CAD build for the part. Positions are in the model's coordinates, mm. Give positions to 0.01 mm unless a question says otherwise; leave off trailing zeros. Put each result on its own line as item: value. Start each with the question number.
1. Drop flat-ended pins along their axis: pin 1 (2 mm diameter, centred on y = -38, z = -75.5, fed in from -X); pin 2 (5 mm diameter, centred on y = -21.5, z = -175.5, fed in from -X); pin 3 (2.5 mm diameter, centred on x = 0, y = -20, fed in from -Z); pin 4 (1.3 mm diameter, centred on x = 1.5, z = -241.5, fed in from -Y). Give the stop position or say it passes through.
2. Cut at A-A on z = -411.5. Give the number of separate pieces and of enclosed holes in the cut face, and give its area (3 significant figures).
3. Wall check: line 1 (Y direction, x = 0, z = -257); line 2 (Y direction, x = -0.5, z = -439.5); line 3 (Y direction, x = 2.5, z = -181). Give the ranges that are in metal, low to high.
from build123d import *

# Parameters (mm, degrees)
SKETCH2_R           = 2.1
BOSS_EXTRUDE2_DEPTH = 500


with BuildPart() as part:
    # Sketch2 → Boss-Extrude2 (new body)
    with BuildSketch(Plane.XY):
        with BuildLine():
            Line((-9.5, 10), (-4.58, 10))
            Line((-4.58, 10), (-3.13, 8.55))
            Line((-3.13, 8.55), (-3.13, 8.2))
            Line((-3.13, 8.2), (-5.5, 8.2))
            Line((-5.5, 8.2), (-5.5, 6.56))
            Line((-5.5, 6.56), (-2.84, 3.9))
            Line((-2.84, 3.9), (-0.21, 3.9))
            Line((-0.21, 3.9), (0, 3.69))
            Line((0, 3.69), (0.21, 3.9))
            Line((0.21, 3.9), (2.84, 3.9))
            Line((2.84, 3.9), (5.5, 6.56))
            Line((5.5, 6.56), (5.5, 8.2))
            Line((5.5, 8.2), (3.13, 8.2))
            Line((3.13, 8.2), (3.13, 8.55))
            Line((3.13, 8.55), (4.58, 10))
            Line((4.58, 10), (9.5, 10))
            ThreePointArc((9.5, 10), (9.853553391, 9.853553391), (10, 9.5))
            Line((10, 9.5), (10, 4.58))
            Line((10, 4.58), (8.55, 3.13))
            Line((8.55, 3.13), (8.2, 3.13))
            Line((8.2, 3.13), (8.2, 5.5))
            Line((8.2, 5.5), (6.56, 5.5))
            Line((6.56, 5.5), (3.9, 2.84))
            Line((3.9, 2.84), (3.9, 0.21))
            Line((3.9, 0.21), (3.69, 0))
            Line((3.69, 0), (3.9, -0.21))
            Line((3.9, -0.21), (3.9, -2.84))
            Line((3.9, -2.84), (6.56, -5.5))
            Line((6.56, -5.5), (8.2, -5.5))
            Line((8.2, -5.5), (8.2, -3.13))
            Line((8.2, -3.13), (8.55, -3.13))
            Line((8.55, -3.13), (10, -4.58))
            Line((10, -4.58), (10, -10))
            Line((10, -10), (10, -15.42))
            Line((10, -15.42), (8.55, -16.87))
            Line((8.55, -16.87), (8.2, -16.87))
            Line((8.2, -16.87), (8.2, -14.5))
            Line((8.2, -14.5), (6.56, -14.5))
            Line((6.56, -14.5), (3.9, -17.16))
            Line((3.9, -17.16), (3.9, -19.79))
            Line((3.9, -19.79), (3.69, -20))
            Line((3.69, -20), (3.9, -20.21))
            Line((3.9, -20.21), (3.9, -22.84))
            Line((3.9, -22.84), (6.56, -25.5))
            Line((6.56, -25.5), (8.2, -25.5))
            Line((8.2, -25.5), (8.2, -23.13))
            Line((8.2, -23.13), (8.55, -23.13))
            Line((8.55, -23.13), (10, -24.58))
            Line((10, -24.58), (10, -30))
            Line((10, -30), (10, -35.42))
            Line((10, -35.42), (8.55, -36.87))
            Line((8.55, -36.87), (8.2, -36.87))
            Line((8.2, -36.87), (8.2, -34.5))
            Line((8.2, -34.5), (6.56, -34.5))
            Line((6.56, -34.5), (3.9, -37.16))
            Line((3.9, -37.16), (3.9, -39.79))
            Line((3.9, -39.79), (3.69, -40))
            Line((3.69, -40), (3.9, -40.21))
            Line((3.9, -40.21), (3.9, -42.84))
            Line((3.9, -42.84), (6.56, -45.5))
            Line((6.56, -45.5), (8.2, -45.5))
            Line((8.2, -45.5), (8.2, -43.13))
            Line((8.2, -43.13), (8.55, -43.13))
            Line((8.55, -43.13), (10, -44.58))
            Line((10, -44.58), (10, -49.5))
            ThreePointArc((10, -49.5), (9.853553391, -49.853553391), (9.5, -50))
            Line((9.5, -50), (4.58, -50))
            Line((4.58, -50), (3.13, -48.55))
            Line((3.13, -48.55), (3.13, -48.2))
            Line((3.13, -48.2), (5.5, -48.2))
            Line((5.5, -48.2), (5.5, -46.56))
            Line((5.5, -46.56), (2.84, -43.9))
            Line((2.84, -43.9), (0.21, -43.9))
            Line((0.21, -43.9), (0, -43.69))
            Line((0, -43.69), (-0.21, -43.9))
            Line((-0.21, -43.9), (-2.84, -43.9))
            Line((-2.84, -43.9), (-5.5, -46.56))
            Line((-5.5, -46.56), (-5.5, -48.2))
            Line((-5.5, -48.2), (-3.13, -48.2))
            Line((-3.13, -48.2), (-3.13, -48.55))
            Line((-3.13, -48.55), (-4.58, -50))
            Line((-4.58, -50), (-9.5, -50))
            ThreePointArc((-9.5, -50), (-9.853553391, -49.853553391), (-10, -49.5))
            Line((-10, -49.5), (-10, -44.58))
            Line((-10, -44.58), (-8.55, -43.13))
            Line((-8.55, -43.13), (-8.2, -43.13))
            Line((-8.2, -43.13), (-8.2, -45.5))
            Line((-8.2, -45.5), (-6.56, -45.5))
            Line((-6.56, -45.5), (-3.9, -42.84))
            Line((-3.9, -42.84), (-3.9, -40.21))
            Line((-3.9, -40.21), (-3.69, -40))
            Line((-3.69, -40), (-3.9, -39.79))
            Line((-3.9, -39.79), (-3.9, -37.16))
            Line((-3.9, -37.16), (-6.56, -34.5))
            Line((-6.56, -34.5), (-8.2, -34.5))
            Line((-8.2, -34.5), (-8.2, -36.87))
            Line((-8.2, -36.87), (-8.55, -36.87))
            Line((-8.55, -36.87), (-10, -35.42))
            Line((-10, -35.42), (-10, -30))
            Line((-10, -30), (-10, -24.58))
            Line((-10, -24.58), (-8.55, -23.13))
            Line((-8.55, -23.13), (-8.2, -23.13))
            Line((-8.2, -23.13), (-8.2, -25.5))
            Line((-8.2, -25.5), (-6.56, -25.5))
            Line((-6.56, -25.5), (-3.9, -22.84))
            Line((-3.9, -22.84), (-3.9, -20.21))
            Line((-3.9, -20.21), (-3.69, -20))
            Line((-3.69, -20), (-3.9, -19.79))
            Line((-3.9, -19.79), (-3.9, -17.16))
            Line((-3.9, -17.16), (-6.56, -14.5))
            Line((-6.56, -14.5), (-8.2, -14.5))
            Line((-8.2, -14.5), (-8.2, -16.87))
            Line((-8.2, -16.87), (-8.55, -16.87))
            Line((-8.55, -16.87), (-10, -15.42))
            Line((-10, -15.42), (-10, -10))
            Line((-10, -10), (-10, -4.58))
            Line((-10, -4.58), (-8.55, -3.13))
            Line((-8.55, -3.13), (-8.2, -3.13))
            Line((-8.2, -3.13), (-8.2, -5.5))
            Line((-8.2, -5.5), (-6.56, -5.5))
            Line((-6.56, -5.5), (-3.9, -2.84))
            Line((-3.9, -2.84), (-3.9, -0.21))
            Line((-3.9, -0.21), (-3.69, 0))
            Line((-3.69, 0), (-3.9, 0.21))
            Line((-3.9, 0.21), (-3.9, 2.84))
            Line((-3.9, 2.84), (-6.56, 5.5))
            Line((-6.56, 5.5), (-8.2, 5.5))
            Line((-8.2, 5.5), (-8.2, 3.13))
            Line((-8.2, 3.13), (-8.55, 3.13))
            Line((-8.55, 3.13), (-10, 4.58))
            Line((-10, 4.58), (-10, 9.5))
            ThreePointArc((-10, 9.5), (-9.853553391, 9.853553391), (-9.5, 10))
        make_face()
        with Locations((0, -20)):
            Circle(SKETCH2_R, mode=Mode.SUBTRACT)
        Circle(SKETCH2_R, mode=Mode.SUBTRACT)
        with Locations((0, -40)):
            Circle(SKETCH2_R, mode=Mode.SUBTRACT)
        Polygon((0.21, -3.9), (0, -3.69), (-0.21, -3.9), (-2.84, -3.9), (-6.24, -7.3), (-8.2, -7.3), (-8.2, -12.7), (-6.24, -12.7), (-2.84, -16.1), (-0.21, -16.1), (0, -16.31), (0.21, -16.1), (2.84, -16.1), (6.24, -12.7), (8.2, -12.7), (8.2, -10), (8.2, -7.3), (6.24, -7.3), (2.84, -3.9), align=None, mode=Mode.SUBTRACT)
        Polygon((-0.21, -36.1), (0, -36.31), (0.21, -36.1), (2.84, -36.1), (6.24, -32.7), (8.2, -32.7), (8.2, -30), (8.2, -27.3), (6.24, -27.3), (2.84, -23.9), (0.21, -23.9), (0, -23.69), (-0.21, -23.9), (-2.84, -23.9), (-6.24, -27.3), (-8.2, -27.3), (-8.2, -32.7), (-6.24, -32.7), (-2.84, -36.1), align=None, mode=Mode.SUBTRACT)
    extrude(amount=-BOSS_EXTRUDE2_DEPTH)


solid = part.part
Report:
1. pin 1: stops at x = -4.06
1. pin 2: stops at x = -9.42
1. pin 3: passes through
1. pin 4: stops at y = -43.9
2. separate pieces: 1
2. enclosed holes: 5
2. area: 428 mm²
3. line 1: y = -43.69 to -42.1, -37.9 to -36.31, -23.69 to -22.1, -17.9 to -16.31, -3.69 to -2.1, 2.1 to 3.69
3. line 2: y = -43.9 to -42.04, -37.96 to -36.1, -23.9 to -22.04, -17.96 to -16.1, -3.9 to -2.04, 2.04 to 3.9
3. line 3: y = -43.9 to -36.1, -23.9 to -16.1, -3.9 to 3.9
